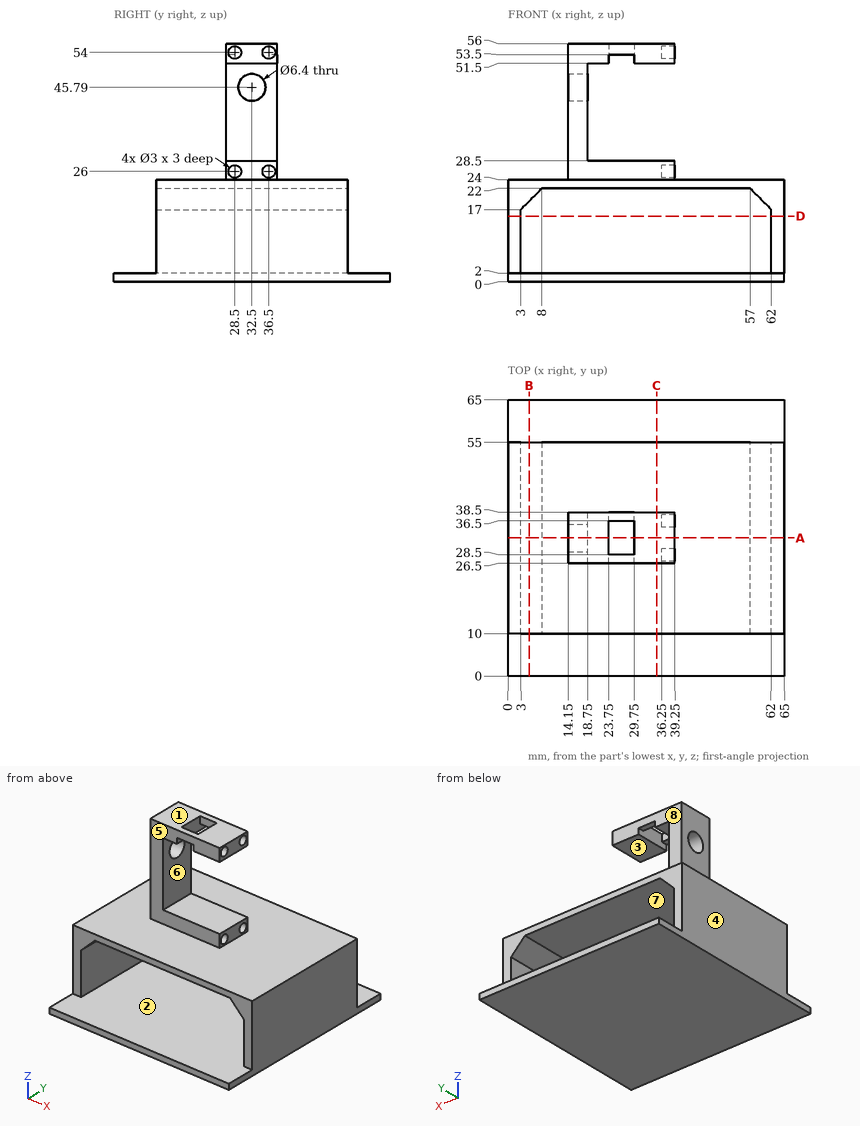
Geometry: see drawing. Coordinates: mm, zero at the bounding-box minimum. A direction names the side the tool comes from. Coordinates: 2 decimals unless noted, no trailing zeros. Order: outer loops, then holes, each group sorted by start corner. A loop starts at its lowest first (then second) coordinate and runs counter-clockwise, first axis right, second up. Notation, with made-up numbers: M 81.25,-15.5 L 88.25,-15.5 A32 ccw 88.25,15.5 Z; hole C 80.5,35.5 d3. An arc over 180 degrees is marked long. Answer in a Markdown table with one row per item. Add a question column.
Q1. Line query: L1, parallel to Y at x = 36.9, z = 26; L2, parallel to Z at x = 37.4, y = 28.5; L3, parallel to Y at x = 15.3, z = 45.79. Output: solid intervals per line, ascending.
Q2. Section query D-D on z = 15.5. Return the cut outline in (x, y).
Q3. Contact query for flat-ended pins moving along their axis: P1, Ø3, axis at y = 12.5, z = 23, coming from the -X side; P2, Ø2, axis at y = 31.5, z = 53.5, coming from the +X side; P3, Ø1, axis at y = 55, z = 25.5, coming from the -X side; P4, Ø3, axis at x = 27.5, z = 54.5, coming from the +Y side. Output: stop coordinate, or through.
Q4. Section query A-A on y = 32.5. Return the cut outline in (x, z).
Q5. Section query B-B on x = 5. Return the cut outline in (y, z).
Q6. Section query C-C on x = 35. Return the cut outline in (y, z), and give its area (3 significant figures).
Q7. Reachability of the marked faces 5, 6, 7 and 8 from +Z, -Z, +X, -X, +Y, -Y: full face, straight path, thin tool, end or side. Return the list, or none.
Q8. Mould query, pull axis Z, two halves, no side actions, for the marked faces 1, 2, 3 and 4. Classes: released by +Z, released by -Z, zero draft, split by the parting line, or undercut.
Completed:
| question | item | result |
|---|---|---|
| 1 | L1 | y = 26.5 to 27, 30 to 35, 38 to 38.5 |
| 1 | L2 | z = 0 to 2, 22 to 24.5, 27.5 to 28.5, 51.5 to 52.5, 55.5 to 56 |
| 1 | L3 | y = 26.5 to 29.3, 35.7 to 38.5 |
| 2 | outline | M 0,10 L 3,10 L 3,55 L 0,55 Z; M 62,10 L 65,10 L 65,55 L 62,55 Z |
| 3 | P1 | stops at x = 0 |
| 3 | P2 | stops at x = 39.25 |
| 3 | P3 | passes through |
| 3 | P4 | stops at y = 38.5 |
| 4 | outline | M 0,0 L 65,0 L 65,24 L 39.25,24 L 39.25,28.5 L 18.75,28.5 L 18.75,42.59 L 14.15,42.59 L 14.15,24 L 0,24 Z; M 14.15,48.99 L 18.75,48.99 L 18.75,51.5 L 23.75,51.5 L 23.75,56 L 14.15,56 Z; M 29.75,51.5 L 39.25,51.5 L 39.25,56 L 29.75,56 Z; hole M 3,2 L 62,2 L 62,17 L 57,22 L 8,22 L 3,17 Z |
| 5 | outline | M 0,0 L 65,0 L 65,2 L 0,2 Z; M 10,19 L 55,19 L 55,24 L 10,24 Z |
| 6 | outline | M 0,0 L 65,0 L 65,2 L 0,2 Z; M 10,22 L 55,22 L 55,24 L 38.5,24 L 38.5,28.5 L 26.5,28.5 L 26.5,24 L 10,24 Z; M 26.5,51.5 L 38.5,51.5 L 38.5,56 L 26.5,56 Z |
| 6 | area | 328 mm2 |
| 7 | face 5 | +Z, +X, -X, -Y |
| 7 | face 6 | +X, +Y, -Y |
| 7 | face 7 | +Y, -Y |
| 7 | face 8 | +Z, +X, -X, +Y |
| 8 | face 1 | released by +Z |
| 8 | face 2 | undercut |
| 8 | face 3 | undercut |
| 8 | face 4 | zero draft |
